Design review of the part shown in the three views and the two pictorial views. Dimensions are in mm from the part's minimum x, y and z. A direction names the side the tool comes from. Coordinates: 2 decimals unless noted, no trailing zeros. Loops run counter-clockwise (first coordinate to the right, second up) from the corner with the lowest first, then second, coordinate; pieces in that order, holes last. Notation, with made-up numbers: (-27.75, 60.5) -> (21.25, 60.5) arc R26 ccw to (21.25, 78.5) -> close; hole circle Ø1 at (-18, 32.5). An arc over 180 degrees is marked (long way). Use a Markdown table: item, result. Add a question column.
Q1. Draft analysis for pull direction Y (two halves, no side actions). For the marked faces 1, 2 and 3, state which applies: pulls with the +Y half, pulls with the -Y half, needs draft (parallel to the pull), parting line crosses it, or undercut.
Q2. For probe 1 along Y at (x, z) = (7, 0.85); probe 2 along Y at (x, z) = (7, 2.4); probe 3 along Y at (x, z) = (2.75, 1.65), list the stretches that pass through material, from the lowest coordinate up.
Q3. Clearance check with flat-ended pins moving along their axes: pin 1 Ø1 at (y, z) = (18.5, 2) entering from -X; pin 2 Ø0.8 at (x, z) = (9.5, 1) entering from +Y; pin 3 Ø1.4 at (x, y) = (7, 19.5) entering from +Z; pin 4 Ø0.6 at (y, z) = (3, 2.5) entering from +X. State where each tip first meets the part, or that it passes through.
Q4. Take a section at C-C on z = 2.5. Write out the cut boundary in (x, y).
Q5. Take a section at A-A on x = 9. Write out the cut boundary in (y, z).
Q6. Take a section at D-D on x = 7. Write out the cut boundary in (y, z).
Q7. For the marked faces 4, 5, 6 and 7, list the 3-axis set-ups (+Z, -Z, +X, -X, +Y, -Y) from which the entire face can be reached by the end or side of a thin tool; tool diameter is ignored.
Q8. Take a section at B-B on y = 9.5. Write out the cut boundary in (x, z), plus the area to 3 significant figures.
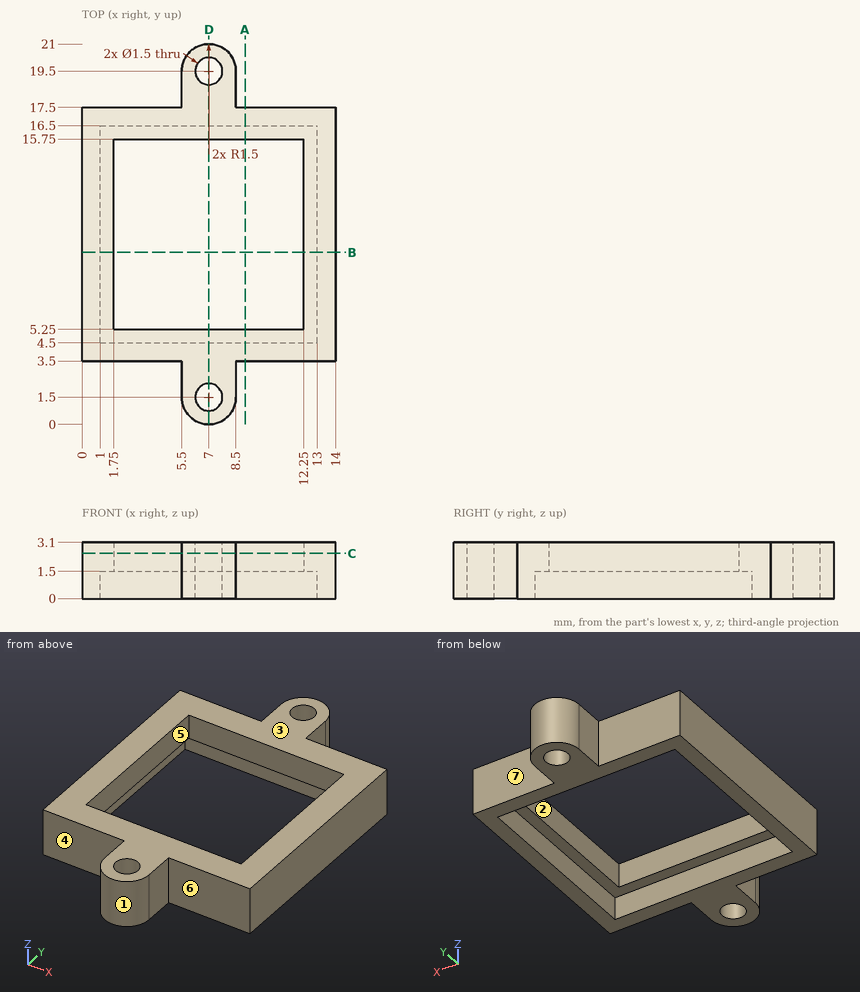
Answer list:
| question | item | result |
|---|---|---|
| 1 | face 1 | pulls with the -Y half |
| 1 | face 2 | undercut |
| 1 | face 3 | needs draft |
| 2 | probe 1 | 0 to 0.75, 2.25 to 4.5, 16.5 to 18.75, 20.25 to 21 |
| 2 | probe 2 | 0 to 0.75, 2.25 to 5.25, 15.75 to 18.75, 20.25 to 21 |
| 2 | probe 3 | 3.5 to 5.25, 15.75 to 17.5 |
| 3 | pin 1 | x = 5.5 |
| 3 | pin 2 | y = 17.5 |
| 3 | pin 3 | through |
| 3 | pin 4 | x = 8.5 |
| 4 | outline | (0, 3.5) -> (5.5, 3.5) -> (5.5, 1.5) arc R1.5 ccw to (8.5, 1.5) -> (8.5, 3.5) -> (14, 3.5) -> (14, 17.5) -> (8.5, 17.5) -> (8.5, 19.5) arc R1.5 ccw to (5.5, 19.5) -> (5.5, 17.5) -> (0, 17.5) -> close; hole (1.75, 5.25) -> (12.25, 5.25) -> (12.25, 15.75) -> (1.75, 15.75) -> close; hole circle Ø1.5 at (7, 1.5); hole circle Ø1.5 at (7, 19.5) |
| 5 | outline | (3.5, 0) -> (4.5, 0) -> (4.5, 1.5) -> (5.25, 1.5) -> (5.25, 3.1) -> (3.5, 3.1) -> close; (15.75, 1.5) -> (16.5, 1.5) -> (16.5, 0) -> (17.5, 0) -> (17.5, 3.1) -> (15.75, 3.1) -> close |
| 6 | outline | (0, 0) -> (0.75, 0) -> (0.75, 3.1) -> (0, 3.1) -> close; (2.25, 0) -> (4.5, 0) -> (4.5, 1.5) -> (5.25, 1.5) -> (5.25, 3.1) -> (2.25, 3.1) -> close; (15.75, 1.5) -> (16.5, 1.5) -> (16.5, 0) -> (18.75, 0) -> (18.75, 3.1) -> (15.75, 3.1) -> close; (20.25, 0) -> (21, 0) -> (21, 3.1) -> (20.25, 3.1) -> close |
| 7 | face 4 | +Z, -Z, -X, -Y |
| 7 | face 5 | +Z, -Z |
| 7 | face 6 | +Z, -Z, +X, -Y |
| 7 | face 7 | +Z, -Z, +X, +Y |
| 8 | outline | (0, 0) -> (1, 0) -> (1, 1.5) -> (1.75, 1.5) -> (1.75, 3.1) -> (0, 3.1) -> close; (12.25, 1.5) -> (13, 1.5) -> (13, 0) -> (14, 0) -> (14, 3.1) -> (12.25, 3.1) -> close |
| 8 | area | 8.60 mm² |
